Drawing for the job (mm, zero at the part's lowest x, y, z). Give positions to 0.01 mm unless a question says otherwise; leave off trailing zeros. Write each loop counter-clockwise with the first axis right and the second up, starting at its lowest first coordinate (ties: lowest second). Pieces come first, ordered by that corner, then holes. Notation, with made-up numbers: (30, 55) - (88, 55) arc R12 cw to (88, 73) - close; hole circle Ø5 at (85.5, 69.5). An arc over 180 degrees is marked (long way). Use CSV: the item, a comma, the result in double quotes.
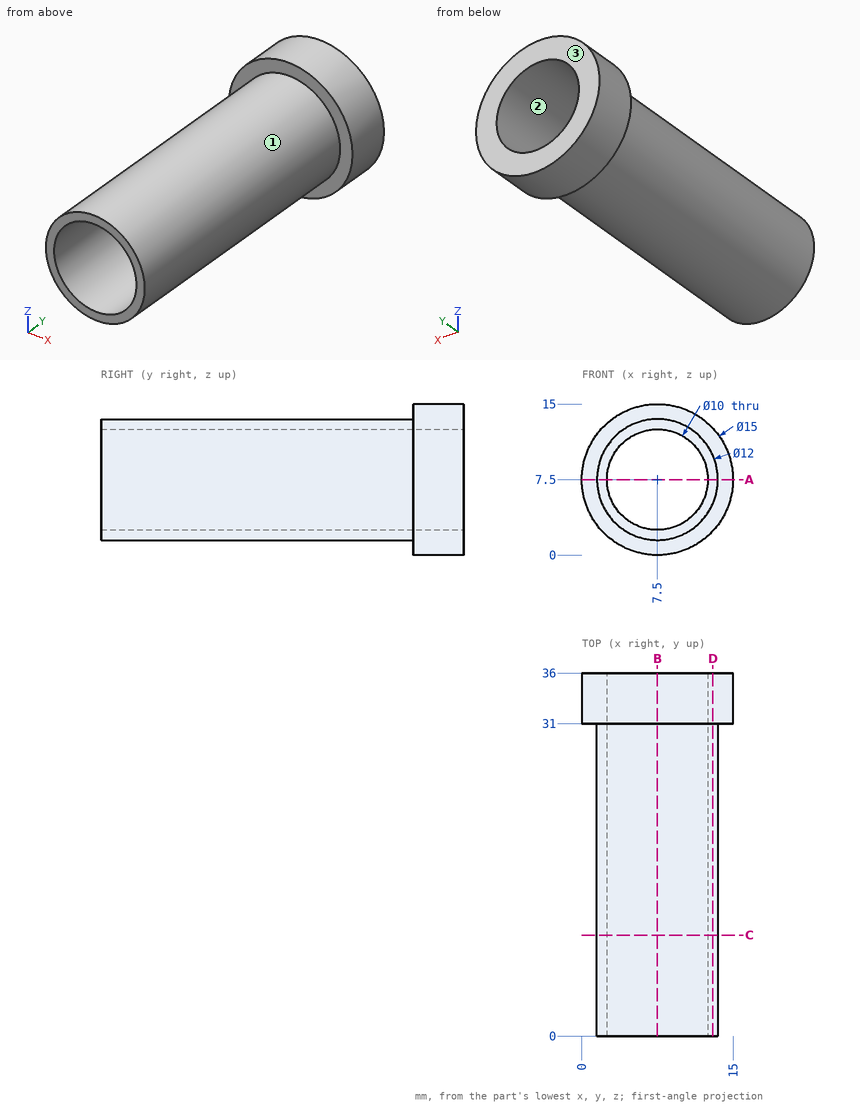
(1) Wall check: probe 1 along Z at (x, y) = (7.5, 21.5); probe 2 along Y at (x, z) = (3, 13); probe 3 along Z at (x, y) = (11, 14). Give the ranges that are in metal, low to high. Write a range as [from, to].
Checked values:
probe 1,"z = [1.5, 2.5], [12.5, 13.5]"
probe 2,"y = [31, 36]"
probe 3,"z = [2.63, 3.93], [11.07, 12.37]"
(2) Saw through at A-A, the plane z = 7.5. List the corners of the cut face in (x, y), then the cut area to 3 significant figures.
Checked values:
outline,"(0, 31) - (1.5, 31) - (1.5, 0) - (2.5, 0) - (2.5, 36) - (0, 36) - close; (12.5, 0) - (13.5, 0) - (13.5, 31) - (15, 31) - (15, 36) - (12.5, 36) - close"
area,"87.0 mm^2"
(3) Saw through at B-B, the plane x = 7.5. List the corners of the cut face in (y, z).
Checked values:
outline,"(0, 1.5) - (31, 1.5) - (31, 0) - (36, 0) - (36, 2.5) - (0, 2.5) - close; (0, 12.5) - (36, 12.5) - (36, 15) - (31, 15) - (31, 13.5) - (0, 13.5) - close"
(4) Pull direction Z, two halves, no side cores. Call the marked faces 1, 2 and 3: released by +Z, released by -Z, zero draft, split by the parting line, or undercut.
Checked values:
face 1,"split by the parting line"
face 2,"undercut"
face 3,"zero draft"
(5) Saw through at D-D, the plane x = 13. List the corners of the cut face in (y, z), then the cut area to 3 significant figures.
Checked values:
outline,"(0, 5.1) - (31, 5.1) - (31, 2.4) - (36, 2.4) - (36, 12.6) - (31, 12.6) - (31, 9.9) - (0, 9.9) - close"
area,"200 mm^2"
(6) Saw through at C-C, the plane y = 10. List the corners of the cut face in (x, z).
Checked values:
outline,"circle Ø12 at (7.5, 7.5); hole circle Ø10 at (7.5, 7.5)"
(7) Flat gauge pins, fed straight in: P1, Ø1, axis at x = 9, y = 26, coming from the +Z side; P2, Ø6, axis at y = 19, z = 12, coming from the -X side; P3, Ø1, axis at x = 6.5, y = 25.5, coming from the -Z side. Where does each tip first touch, or does it go through?
Checked values:
P1,"stops at z = 13.42"
P2,"stops at x = 1.69"
P3,"stops at z = 1.52"
